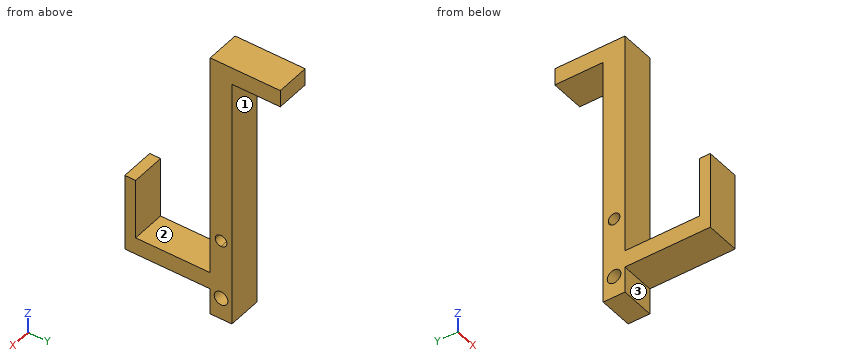
from build123d import *

# Parameters (mm, degrees)
SKETCH1_W           = 5
SKETCH1_H           = 14.17103806
BOSS_EXTRUDE1_DEPTH = 10


with BuildPart() as part:
    # Sketch1 → Boss-Extrude1 (new body)
    with BuildSketch(Plane(origin=(0, 0, 0), x_dir=(0, 0, -1), z_dir=(1, 0, 0))):
        with BuildLine():
            Line((-61.2, 21.825), (-6.35, 21.825))
            Line((-6.35, 21.825), (-6.35, 23.3))
            ThreePointArc((-6.35, 23.3), (-8.05, 25), (-6.35, 26.7))
            Line((-6.35, 26.7), (-6.35, 28.175))
            Line((-6.35, 28.175), (-56.2, 28.175))
            Line((-56.2, 28.175), (-61.2, 28.175))
            Line((-61.2, 28.175), (-61.2, 21.825))
        make_face()
        with BuildLine():
            Line((-6.35, 21.825), (0, 21.825))
            Line((0, 21.825), (5, 21.825))
            Line((5, 21.825), (10, 21.825))
            Line((10, 21.825), (17.7, 21.825))
            Line((17.7, 21.825), (17.7, 25))
            Line((17.7, 25), (13.35, 25))
            ThreePointArc((13.35, 25), (11.35, 23), (9.35, 25))
            Line((9.35, 25), (-4.65, 25))
            ThreePointArc((-4.65, 25), (-5.147918472, 23.797918472), (-6.35, 23.3))
            Line((-6.35, 23.3), (-6.35, 21.825))
        make_face()
        with BuildLine():
            Line((-6.35, 28.175), (-6.35, 26.7))
            ThreePointArc((-6.35, 26.7), (-5.147918472, 26.202081528), (-4.65, 25))
            Line((-4.65, 25), (9.35, 25))
            ThreePointArc((9.35, 25), (11.35, 27), (13.35, 25))
            Line((13.35, 25), (17.7, 25))
            Line((17.7, 25), (17.7, 28.175))
            Line((17.7, 28.175), (-6.35, 28.175))
        make_face()
        Polygon((5, 21.825), (5, 0), (5, -3.175), (10, -3.175), (10, 21.825), align=None)
        Polygon((5, 0), (0, 0), (-12.7, 0), (-12.7, -3.175), (5, -3.175), align=None)
        with Locations((-58.7, 35.26051903)):
            Rectangle(SKETCH1_W, SKETCH1_H)
    extrude(amount=BOSS_EXTRUDE1_DEPTH)


solid = part.part
Could you check a few things on this model? Use its own coordinates, in mm. Face numbers are marked on the shaded views. A direction names the side the tool comes from. Coordinates: 2 decimals unless noted, no trailing zeros. Order: outer loops, then holes, each group sorted by start corner. A loop starts at its lowest first (then second) coordinate and runs counter-clockwise, first axis right, second up. Notation, with made-up numbers: (-10, 72) - (-2, 72) arc R13 ccw to (-2, 93) - close; hole circle Ø10 at (-8, 35). An arc over 180 degrees is marked (long way). Answer in a Markdown table with one row per item. Add a question column.
(1) If we section it at A-A, the plane z = -11.35: Please give me the cut outline in (x, y) (3 decimals).
(2) On a 3-axis mill with a long thin cutter (end or side, diameter ignored), from which of +Z, -Z, +X, -X, +Y, -Y can I reach the whole of each face in a straight line? I mean the marked faces 1, 2 and 3. Say none if no direction works.
(3) Will these pins go through, and if not, where does the flat tip stop? pin 1 (1 mm diameter, centred on x = 6, y = 32, fed in from -Z); pin 2 (1 mm diameter, centred on x = 2, z = 52.5, fed in from +Y) (3 decimals); pin 3 (5 mm diameter, centred on y = 25, z = -11.35, fed in from -X); pin 4 (4 mm diameter, centred on x = 3.5, z = -12.5, fed in from -Y) (3 decimals).
(4) If we section it at C-C, the plane y = 1: Please give me the cut outline in (x, z), then the cut area to 3 significant figures.
(5) If we section it at D-D, the plane z = 30.5: Please give me the cut outline in (x, y) (3 decimals).
(6) If we section it at B-B, the plane x = 1: Please give me the cut outline in (y, z) (3 decimals).
(7) I need wall thicknesses on L1, parallel to Y at x = 2.5, z = -11.35 (3 decimals); L2, parallel to Y at x = 4.25, z = 11.5 (3 decimals); L3, parallel to Y at x = 9.25, z = 7.5 (3 decimals). Which ranges of each line are inside material? Lowest first, please.
Results are:
| question | item | result |
|---|---|---|
| 1 | outline | (0, 21.825) - (10, 21.825) - (10, 23) - (0, 23) - close; (0, 27) - (10, 27) - (10, 28.175) - (0, 28.175) - close |
| 2 | face 1 | -Z, +X, -X, +Y |
| 2 | face 2 | +Z, +X, -X |
| 2 | face 3 | -Z, +X, -X, -Y |
| 3 | pin 1 | stops at z = 56.2 |
| 3 | pin 2 | stops at y = 28.175 |
| 3 | pin 3 | stops at x = 0 |
| 3 | pin 4 | stops at y = 21.825 |
| 4 | outline | (0, -10) - (10, -10) - (10, -5) - (0, -5) - close |
| 4 | area | 50.0 mm2 |
| 5 | outline | (0, 21.825) - (10, 21.825) - (10, 28.175) - (0, 28.175) - close |
| 6 | outline | (-3.175, -10) - (21.825, -10) - (21.825, -17.7) - (28.175, -17.7) - (28.175, 56.2) - (42.346, 56.2) - (42.346, 61.2) - (21.825, 61.2) - (21.825, -5) - (0, -5) - (0, 12.7) - (-3.175, 12.7) - close; hole circle Ø4 at (25, -11.35); hole circle Ø3.4 at (25, 6.35) |
| 7 | L1 | y = 21.825 to 23, 27 to 28.175 |
| 7 | L2 | y = -3.175 to 0, 21.825 to 28.175 |
| 7 | L3 | y = -3.175 to 0, 21.825 to 23.748, 26.252 to 28.175 |
